The listing builds one solid part. Answer for the finished solid, in the listing's coordinates (mm). Face numbers are marked on the shaded views. A direction names the side the tool comes from. Coordinates: 2 decimals unless noted, no trailing zeros. Write each loop counter-clockwise with the first axis right and the second up, starting at its lowest first coordinate (ties: lowest second). Pieces come first, ordered by that corner, then holes. Notation, with made-up numbers: M 62,56 L 113,56 A16 cw 113,70 Z; hole C 59.5,0 d8. An arc over 180 degrees is marked long. Answer as CSV lines item,"result". Start each with the question number.
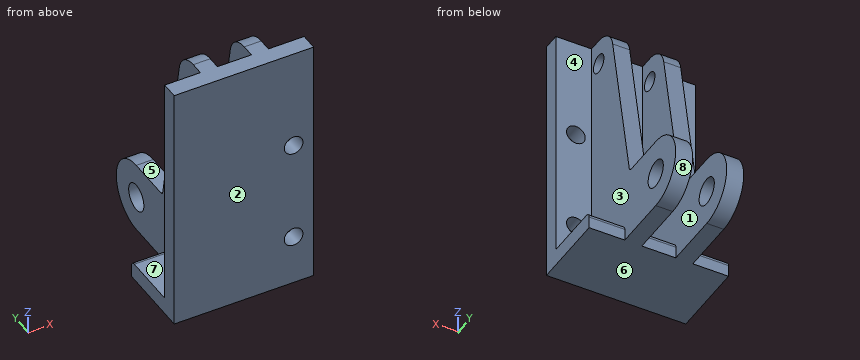
```python
from build123d import *

# Parameters (mm, degrees)
BOSS_EXTRUDE1_DEPTH = 82
SKETCH2_R           = 8
SKETCH2_R_2         = 5.5
BOSS_EXTRUDE2_DEPTH = 10
SKETCH3_R           = 5.5
CUT_EXTRUDE1_DEPTH  = 148.200134968


with BuildPart() as part:
    # Sketch1 → Boss-Extrude1 (new body)
    with BuildSketch(Plane(origin=(0, 0, 0), x_dir=(0, 0, -1), z_dir=(1, 0, 0))):
        with BuildLine():
            Line((-84.297520661, 0), (65.702479339, 0))
            Line((65.702479339, 0), (65.702479339, 45))
            Line((65.702479339, 45), (58.702479339, 45))
            ThreePointArc((58.702479339, 45), (56.581158995, 44.121320344), (55.702479339, 42))
            Line((55.702479339, 42), (55.702479339, 10))
            Line((55.702479339, 10), (-84.297520661, 10))
            Line((-84.297520661, 10), (-84.297520661, 0))
        make_face()
    extrude(amount=-BOSS_EXTRUDE1_DEPTH)

    # Sketch2 → Boss-Extrude2 (add)
    with BuildSketch(Plane(origin=(-21, 0, 0), x_dir=(0, 0, -1), z_dir=(1, 0, 0))):
        with BuildLine():
            Line((65.702479339, 45), (65.702479339, 77.531394121))
            ThreePointArc((65.702479339, 77.531394121), (44.702479339, 98.531394121), (23.702479339, 77.531394121))
            Line((23.702479339, 77.531394121), (23.702479339, 51.663245522))
            ThreePointArc((23.702479339, 51.663245522), (23.240214757, 50.384429748), (22.067109554, 49.696765213))
            Line((22.067109554, 49.696765213), (-72.032247278, 32.248602318))
            ThreePointArc((-72.032247278, 32.248602318), (-80.830536296, 27.091118307), (-84.297520661, 17.5))
            Line((-84.297520661, 17.5), (-84.297520661, 10))
            Line((-84.297520661, 10), (55.702479339, 10))
            Line((55.702479339, 10), (55.702479339, 42))
            ThreePointArc((55.702479339, 42), (56.581158995, 44.121320344), (58.702479339, 45))
            Line((58.702479339, 45), (65.702479339, 45))
        make_face()
        with Locations((44.702479339, 77.531394121)):
            Circle(SKETCH2_R, mode=Mode.SUBTRACT)
        with Locations((-69.297520661, 17.5)):
            Circle(SKETCH2_R_2, mode=Mode.SUBTRACT)
    extrude(amount=-BOSS_EXTRUDE2_DEPTH)

    # Mirror1: part across plane


with BuildPart() as part_1:
    add(part.part)
    add(part.part.mirror(Plane(origin=(-41, 0, 0), x_dir=(0, 0, 1), z_dir=(1, 0, 0))))

    # Sketch3 → Cut-Extrude1 (cut, through all)
    with BuildSketch(Plane(origin=(0, 10, 0), x_dir=(1, 0, 0), z_dir=(0, 1, 0))):
        with Locations(Location((-11.776828818, -24.297520661, 0), (0, 0, 270))):
            Circle(SKETCH3_R)
        with Locations(Location((-11.776828818, 35.702479339, 0), (0, 0, 270))):
            Circle(SKETCH3_R)
    extrude(amount=-CUT_EXTRUDE1_DEPTH, mode=Mode.SUBTRACT)


solid = part_1.part
```
1) The part is cut by section B-B (y = 64). Determine the outline of the cut face in (x, z).
2) The part is cut by section C-C (x = -75.5). Determine the outline of the cut face in (y, z).
3) Each of these flat-tipped pins is pushed along its axis until it touches: P1, Ø3.5, axis at x = -42, z = -61.5, coming from the +Y side; P2, Ø5, axis at x = -25, y = 64.5, coming from the +Z side; P3, Ø1, axis at y = 26.5, z = -21, coming from the +X side; P4, Ø10, axis at y = 17.5, z = 69.3, coming from the +X side. Where does it stop, or does it pass through?
4) The part is cut by section A-A (z = -35). Determine the outline of the cut face in (x, y).
5) The part is cut by section D-D (y = 74). Determine the outline of the cut face in (x, z), then the cut area to 3 significant figures.
6) For a pull along X with two mould halves and no side action, classify the marked faces 1, 2 and 3 as +X half, -X half, draft (parallel to the pull), parting line (faces both ways), or undercut.
7) Which of the six approach directions +Z, -Z, +X, -X, +Y, -Y give full straight-line access (tool end or side, diameter ignored) to the marked faces 4, 5, 6, 7 and 8?
8) Find the intervals of material crossed by line 1 (X direction, y = 26.5, z = -33); line 2 (Y direction, x = -70.5, z = 8); line 3 (Y direction, x = -35, z = -59), in increasing order. Write a range as from..to.
Completed:
1,outline,"M -61,-65.7 L -51,-65.7 L -51,-23.7 L -61,-23.7 Z; M -31,-65.7 L -21,-65.7 L -21,-23.7 L -31,-23.7 Z"
2,outline,"M 0,-65.7 L 45,-65.7 L 45,-58.7 A3 ccw 42,-55.7 L 10,-55.7 L 10,84.3 L 0,84.3 Z"
3,P1,"y = 45"
3,P2,"z = -23.7"
3,P3,"x = -21"
3,P4,"through"
4,outline,"M -82,0 L -17.23,0 L -17.23,10 L -21,10 L -21,96.16 L -31,96.16 L -31,10 L -51,10 L -51,96.16 L -61,96.16 L -61,10 L -82,10 Z; M -6.32,0 L 0,0 L 0,10 L -6.32,10 Z"
5,outline,"M -61,-65.7 L -51,-65.7 L -51,-51.88 L -61,-51.88 Z; M -61,-37.52 L -51,-37.52 L -51,-23.7 L -61,-23.7 Z; M -31,-65.7 L -21,-65.7 L -21,-51.88 L -31,-51.88 Z; M -31,-37.52 L -21,-37.52 L -21,-23.7 L -31,-23.7 Z"
5,area,"553 mm²"
6,face 1,"undercut"
6,face 2,"draft"
6,face 3,"+X half"
7,face 4,"+Z, +X, +Y"
7,face 5,"+Z, +X, -X, +Y"
7,face 6,"-Z, +X, -X, +Y, -Y"
7,face 7,"+Z, -X, +Y"
7,face 8,"+X, -X, +Y"
8,line 1,"-61..-51, -31..-21"
8,line 2,"0..10"
8,line 3,"0..45"
